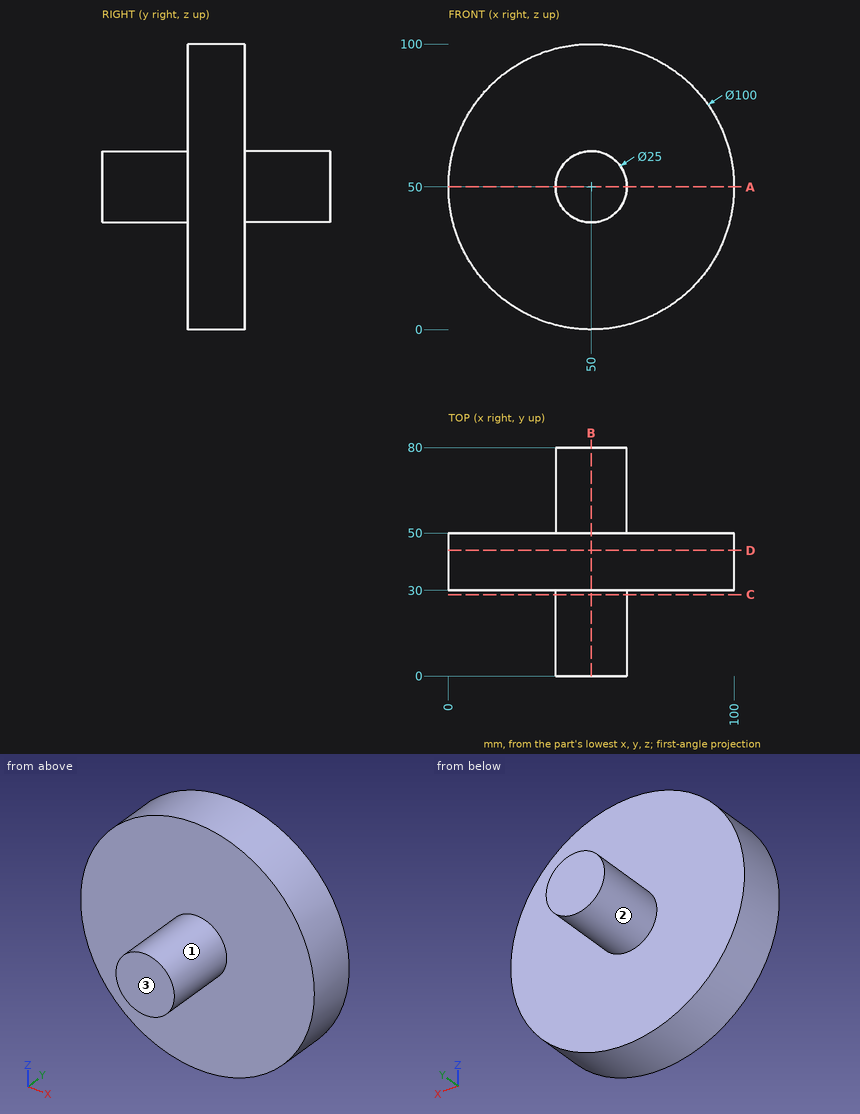
Source: three-view drawing plus pictorial views. Frame: mm from the lowest corner of the part. A direction names the side the tool comes from. Round coordinates to 2 decimals unless told otherwise and drop trailing zeros. Order: outer loops, then holes, each group sorted by start corner. A loop starts at its lowest first (then second) coordinate and runs counter-clockwise, first axis right, second up. Notation, with made-up numbers: (46, -11) -> (103, -11) arc R30 ccw to (103, 12) -> close; hole circle Ø8 at (42.5, 0.5). An arc over 180 degrees is marked (long way). Use one line per item in the form item = value. Start each with the question number.
1. Line query: probe 1 along Y at (x, z) = (24, 89); probe 2 along Z at (x, y) = (41, 67); probe 3 along X at (y, z) = (41, 37). Output: solid intervals per line, ascending.
2. Cut plane A-A (z = 50). Return the cut outline in (x, y), then the cut area to 3 significant figures.
3. Cut plane C-C (y = 28.5). Return the cut outline in (x, z).
4. Reachability of the marked faces 1, 2 and 3 from +Z, -Z, +X, -X, +Y, -Y: full face, straight path, thin tool, end or side. Return the list, or none.
5. Pin query (flat end, axial travel): pin 1 Ø10 at (y, z) = (45.5, 81.5) entering from -X; pin 2 Ø10 at (x, z) = (47.5, 80.5) entering from -Y; pin 3 Ø1 at (y, z) = (41.5, 72.5) entering from +X; pin 4 Ø2 at (x, z) = (10.5, 17) entering from +Y. Return the tip coordinate at first contact, or that it passes through.
6. Cut plane B-B (x = 50). Return the cut outline in (y, z), then the cut area to 3 significant figures.
7. Cut plane D-D (y = 44). Return the cut outline in (x, z), then the cut area to 3 significant figures.
Solution:
q1.probe_1 = 30 to 50
q1.probe_2 = 41.33 to 58.67
q1.probe_3 = 1.72 to 98.28
q2.outline = (0, 30) -> (37.5, 30) -> (37.5, 0) -> (62.5, 0) -> (62.5, 30) -> (100, 30) -> (100, 50) -> (62.5, 50) -> (62.5, 80) -> (37.5, 80) -> (37.5, 50) -> (0, 50) -> close
q2.area = 3,500 mm^2
q3.outline = circle Ø25 at (50, 50)
q4.face_1 = -Y
q4.face_2 = +Y
q4.face_3 = +Z, -Z, +X, -X, -Y
q5.pin_1 = 7.6
q5.pin_2 = 30
q5.pin_3 = 94.9
q5.pin_4 = through
q6.outline = (0, 37.5) -> (30, 37.5) -> (30, 0) -> (50, 0) -> (50, 37.5) -> (80, 37.5) -> (80, 62.5) -> (50, 62.5) -> (50, 100) -> (30, 100) -> (30, 62.5) -> (0, 62.5) -> close
q6.area = 3,500 mm^2
q7.outline = circle Ø100 at (50, 50)
q7.area = 7,850 mm^2
